Could you check a few things on this drawing? It's one solid part, dimensions in mm from its lowest x, y, z. A direction names the side the tool comes from. Coordinates: 2 decimals unless noted, no trailing zeros. Order: outer loops, then holes, each group sorted by start corner. A loop starts at its lowest first (then second) coordinate and runs counter-clockwise, first axis right, second up.
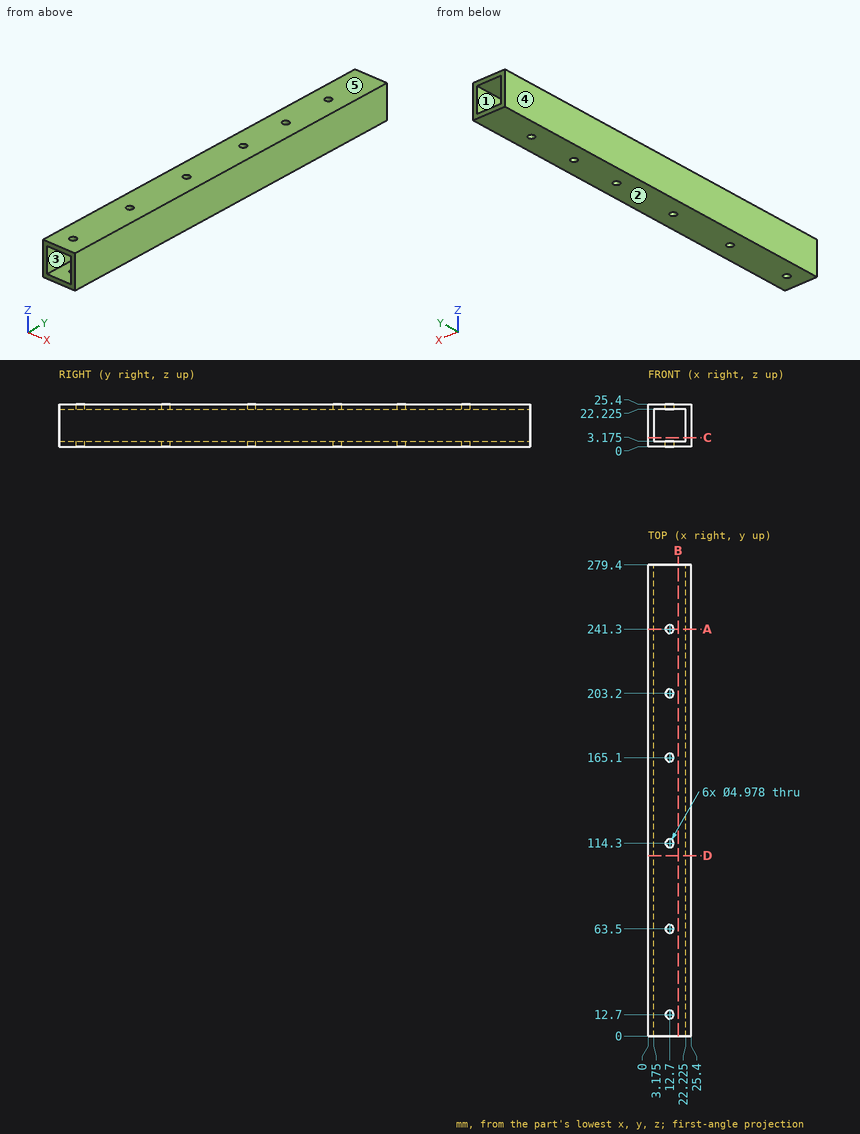
Item 1: For pin 1 Ø8 at (x, y) = (12.7, 12.7) entering from -Z, with a flat end and sliding along its axis, tell me the tip position at first contact or that it passes through.
Item 2: Thinking about a two-plate mould opening in X: for the marked faces 3, 4 and 5, which applies, +X half, -X half, draft (parallel to the pull), parting line (faces both ways), or undercut?
Item 3: Suppose I cut it at D-D (y = 107). List the corners of the cut face in (x, z) for me (1 decimal), and give its area (3 significant figures).
Item 4: Suppose I cut it at C-C (z = 5.5). List the corners of the cut face in (x, y) for me (1 decimal).
Item 5: Which directions (+Z, -Z, +X, -X, +Y, -Y) give clear straight access to the entire face, cutting with the end or side of a thin tool? Please do the marked faces 1 and 2.
Item 6: Suppose I cut it at A-A (y = 241.3). List the corners of the cut face in (x, z) for me (1 decimal), and give its area (3 significant figures).
Item 7: I need wall thicknesses on line 1 (Z direction, x = 21, y = 199) (1 decimal). Which ranges of the line are inside material? Lowest first, please.
Item 8: Suppose I cut it at B-B (x = 17.75). List the corners of the cut face in (y, z) for me (1 decimal).
Geometry results:
1. pin 1: stops at z = 0
2. face 3: undercut
2. face 4: -X half
2. face 5: draft
3. outline: (0, 0) - (25.4, 0) - (25.4, 25.4) - (0, 25.4) - close; hole (3.2, 3.2) - (22.2, 3.2) - (22.2, 22.2) - (3.2, 22.2) - close
3. area: 282 mm2
4. outline: (0, 0) - (3.2, 0) - (3.2, 279.4) - (0, 279.4) - close; (22.2, 0) - (25.4, 0) - (25.4, 279.4) - (22.2, 279.4) - close
5. face 1: +Y, -Y
5. face 2: -Z, +X, -X, +Y, -Y
6. outline: (0, 0) - (10.2, 0) - (10.2, 3.2) - (3.2, 3.2) - (3.2, 22.2) - (10.2, 22.2) - (10.2, 25.4) - (0, 25.4) - close; (15.2, 0) - (25.4, 0) - (25.4, 25.4) - (15.2, 25.4) - (15.2, 22.2) - (22.2, 22.2) - (22.2, 3.2) - (15.2, 3.2) - close
6. area: 251 mm2
7. line 1: z = 0 to 3.2, 22.2 to 25.4
8. outline: (0, 0) - (279.4, 0) - (279.4, 3.2) - (0, 3.2) - close; (0, 22.2) - (279.4, 22.2) - (279.4, 25.4) - (0, 25.4) - close
